For this review, take the finished solid that the model builds, in its own axes (mm). A direction names the side the tool comes from. Round coordinates to 2 decimals unless told otherwise and drop trailing zeros. Write each loop counter-clockwise with the first axis right and the second up, starting at its lowest first coordinate (ties: lowest second). Pieces come first, ordered by that corner, then holes.
from build123d import *

# Parameters (mm, degrees)
F0_R     = 22.5
F0_R_2   = 18
F1_DEPTH = 3
F2_R     = 30
F2_R_2   = 2.25
F3_DEPTH = 6
F4_DEPTH = 3
F5_R     = 10
F6_DEPTH = 10


with BuildPart() as f1:
    # F0 (on Top) → F1 (new body)
    with BuildSketch(Plane.XY):
        with Locations((-35.527975389, 25.6118375491)):
            Circle(F0_R)
        with Locations((-35.527975389, 25.6118375491)):
            Circle(F0_R_2, mode=Mode.SUBTRACT)
    extrude(amount=F1_DEPTH)


with BuildPart() as f3:
    # F2 (on Top) → F3 (new body)
    with BuildSketch(Plane.XY):
        with Locations((-35.527975389, 25.6118375491)):
            Circle(F2_R)
        with Locations((-51.7297042582, 3.6392641531)):
            Circle(F2_R_2, mode=Mode.SUBTRACT)
        with Locations((-41.3919404606, -1.0509438819)):
            Circle(F2_R_2, mode=Mode.SUBTRACT)
        with Locations((-59.2660419463, 12.1287297427)):
            Circle(F2_R_2, mode=Mode.SUBTRACT)
        with Locations((-62.697852273, 22.9495471623)):
            Circle(F2_R_2, mode=Mode.SUBTRACT)
        with Locations((-30.0402438296, -1.1309147837)):
            Circle(F2_R_2, mode=Mode.SUBTRACT)
        with Locations((-19.6374258397, 3.4131791432)):
            Circle(F2_R_2, mode=Mode.SUBTRACT)
        with Locations((-11.982228228, 11.7956227769)):
            Circle(F2_R_2, mode=Mode.SUBTRACT)
        with Locations((-8.3983042068, 22.5670154611)):
            Circle(F2_R_2, mode=Mode.SUBTRACT)
        with Locations((-61.4317440559, 34.230698776)):
            Circle(F2_R_2, mode=Mode.SUBTRACT)
        with Locations((-55.686638908, 44.0215709836)):
            Circle(F2_R_2, mode=Mode.SUBTRACT)
        with Locations((-46.4559177018, 50.6292330332)):
            Circle(F2_R_2, mode=Mode.SUBTRACT)
        with Locations((-9.5053467983, 33.8648855457)):
            Circle(F2_R_2, mode=Mode.SUBTRACT)
        with Locations((-35.3356559926, 52.9111601277)):
            Circle(F2_R_2, mode=Mode.SUBTRACT)
        with Locations((-24.2486480541, 50.4727863418)):
            Circle(F2_R_2, mode=Mode.SUBTRACT)
        with Locations((-15.1119382813, 43.7357286551)):
            Circle(F2_R_2, mode=Mode.SUBTRACT)
    extrude(amount=F3_DEPTH)


with BuildPart() as f4_tool:
    # F0 (on Top) → F4 (new body)
    with BuildSketch(Plane.XY):
        with Locations((-35.527975389, 25.6118375491)):
            Circle(F0_R)
        with Locations((-35.527975389, 25.6118375491)):
            Circle(F0_R_2, mode=Mode.SUBTRACT)
    extrude(amount=F4_DEPTH)


with BuildPart() as f1_1:
    add(f1.part)

    # F4: cut by f4_tool
    add(f4_tool.part, mode=Mode.SUBTRACT)


with BuildPart() as f3_1:
    add(f3.part)

    # F4: cut by f4_tool
    add(f4_tool.part, mode=Mode.SUBTRACT)

    # F5 (on face) → F6 (cut)
    with BuildSketch(Plane(origin=(0, 0, 0), x_dir=(1, 0, 0), z_dir=(0, 0, -1))):
        with Locations((-35.527975389, -25.6118375491)):
            Circle(F5_R)
    extrude(amount=-F6_DEPTH, mode=Mode.SUBTRACT)


solid = f3_1.part
(1) We need section B-B, the plane x = -20.5. Give the boundary of the cut face in (y, z), and give its area (3 significant figures).
Geometry check:
outline: (-0.35, 0) - (1.34, 0) - (1.34, 6) - (-0.35, 6) - close; (5.49, 0) - (8.87, 0) - (8.87, 3) - (15.7, 3) - (15.7, 0) - (35.52, 0) - (35.52, 3) - (42.36, 3) - (42.36, 0) - (51.58, 0) - (51.58, 6) - (5.49, 6) - close
area: 246 mm2
(2) We need section A-A, the plane y = 30. Give the boundary of the cut face in (x, z).
Geometry check:
outline: (-65.21, 0) - (-57.6, 0) - (-57.6, 3) - (-52.98, 3) - (-52.98, 0) - (-44.51, 0) - (-44.51, 6) - (-65.21, 6) - close; (-26.54, 0) - (-18.07, 0) - (-18.07, 3) - (-13.46, 3) - (-13.46, 0) - (-5.85, 0) - (-5.85, 6) - (-26.54, 6) - close
(3) For pin 1 Ø4 at (x, y) = (-61.43, 34.23) entering from +Z; pin 2 Ø1 at (y, z) = (19, 2.5) entering from -X; pin 3 Ø1 at (x, y) = (-26.5, 7.5) entering from -Z; pin 4 Ø1 at (y, z) = (32, 5) entering from +X, all flat-tipped, find the tip position at first contact; note any pin that passes through.
Geometry check:
pin 1: passes through
pin 2: stops at x = -64.9
pin 3: stops at z = 3
pin 4: stops at x = -6.11
(4) Mouldability with a two-part tool opening along X and no side actions: class faces 1 (the face through (-21.68, -1, 2.96)), 2 (the face through (-49.812, 14.659, 1.479)), 3 (the face through (-40, 48, 0)) as pulls with the +X half, pulls with the -X half, needs draft (parallel to the pull), parting line crosses it, or undercut.
Geometry check:
face 1: parting line crosses it
face 2: undercut
face 3: needs draft
(5) We need section C-C, the plane z = 4.8. State how many separate pieces and enclosed holes the cut face has, and give its area (3 significant figures).
Geometry check:
separate pieces: 1
enclosed holes: 16
area: 2,270 mm2
(6) We need section D-D, the plane y = 0. Give the boundary of the cut face in (x, z), and give its area (3 significant figures).
Geometry check:
outline: (-51.15, 0) - (-43.38, 0) - (-43.38, 6) - (-51.15, 6) - close; (-39.4, 0) - (-31.99, 0) - (-31.99, 6) - (-39.4, 6) - close; (-28.1, 0) - (-19.91, 0) - (-19.91, 6) - (-28.1, 6) - close
area: 140 mm2
(7) For faces 4 (the face through (-59.353, 33.369, 2.958)), 5 (the face through (-46, 41, 3)), list the 3-axis set-ups (+Z, -Z, +X, -X, +Y, -Y) from which the entire face can be reached by the end or side of a thin tool; tool diameter is ignored.
Geometry check:
face 4: +Z, -Z
face 5: -Z
(8) For line 1 along Y through (x, z) = (-51, 0.25); line 2 along X through (y, z) = (52, 3.3); line 3 along X through (y, z) = (45.5, 4.1), list the stretches that pass through material, from the lowest coordinate up.
Geometry check:
line 1: y = -0.09 to 1.51, 5.77 to 9.28, 16.41 to 34.81, 41.95 to 51.31
line 2: x = -49.8 to -48.24, -44.67 to -37.39, -33.28 to -25.9, -22.6 to -21.26
line 3: x = -57.99 to -57.38, -53.99 to -16.51, -13.72 to -13.07
